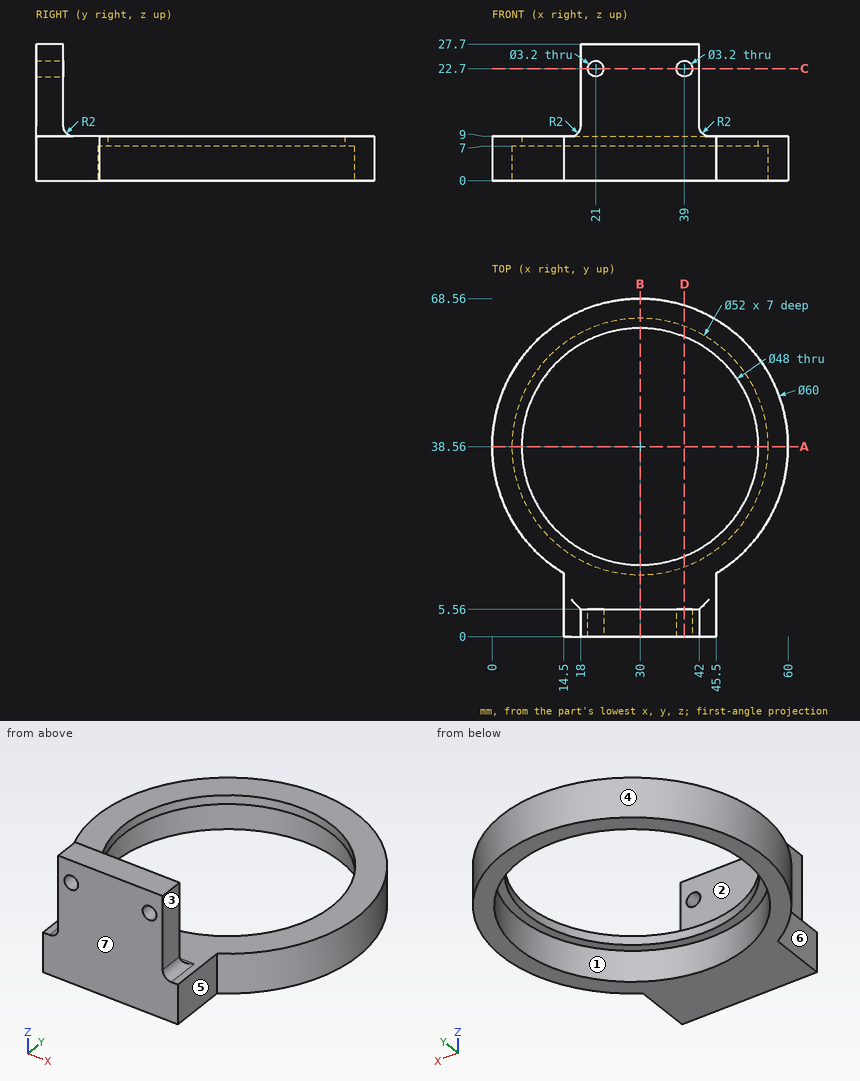
Study the drawing (mm; zero at the part's minimum x, y, z) and answer. A direction names the side the tool comes from. Give positions to 0.01 mm unless a question says otherwise; leave off trailing zeros. Write each loop counter-clockwise with the first axis right and the second up, starting at its lowest first coordinate (ties: lowest second). Pieces come first, ordered by that corner, then holes. Notation, with made-up numbers: (59, 78) -> (67, 78) arc R15 cw to (67, 105) -> close; hole circle Ø9 at (66.5, 70). An arc over 180 degrees is marked (long way). Answer as a JSON object with one key per item and string values. Group by question number.
1) Each of these flat-tipped pins is pushed along its axis until it touches: P1, Ø4.5, axis at y = 1.5, z = 20, coming from the +X side; P2, Ø7, axis at y = 8.5, z = 6, coming from the -X side; P3, Ø3, axis at y = 2.5, z = 19.5, coming from the -X side. Where does it stop, or does it pass through?
2) Find section B-B (x = 30). Write down the section's boundary in (y, z).
3) The mould has two halves that part along Y. Classify the marked faces 1, 2, 3 and 4: +Y half, -Y half, draft (parallel to the pull), parting line (faces both ways), or undercut.
4) Find section D-D (x = 39). Write down the section's boundary in (y, z), and give its area (3 significant figures).
5) Find section A-A (y = 38.56). Write down the section's boundary in (x, z), and give its area (3 significant figures).
6) Consider L1, parallel to X at y = 2.65, z = 22.7; L2, parallel to Z at x = 39, y = 3; L3, parallel to Y at x = 30, z = 3.75. Determine where each line is inside the solid, lowest interval first. Write a range as from..to.
7) A tool of negligible diameter and unlimited length cuts with its end or side. For the marked faces 5, 6 and 7, from which of +Z, -Z, +X, -X, +Y, -Y can it reach the whole face along a straight path? Write none if from no direction.
8) Find section C-C (z = 22.7). Write down the section's boundary in (x, y), and give its area (3 significant figures).
Values follow:
{
 "1": {"P1": "stops at x = 42", "P2": "stops at x = 14.5", "P3": "stops at x = 18"},
 "2": {"outline": "(0, 0) -> (12.56, 0) -> (12.56, 7) -> (14.56, 7) -> (14.56, 9) -> (7.56, 9) arc R2 cw to (5.56, 11) -> (5.56, 27.7) -> (0, 27.7) -> close; (62.56, 7) -> (64.56, 7) -> (64.56, 0) -> (68.56, 0) -> (68.56, 9) -> (62.56, 9) -> close"},
 "3": {"face 1": "undercut", "face 2": "+Y half", "face 3": "draft", "face 4": "parting line"},
 "4": {"outline": "(0, 0) -> (14.17, 0) -> (14.17, 7) -> (16.31, 7) -> (16.31, 9) -> (7.56, 9) arc R2 cw to (5.56, 11) -> (5.56, 21.1) -> (0, 21.1) -> close; (0, 24.3) -> (5.56, 24.3) -> (5.56, 27.7) -> (0, 27.7) -> close; (60.81, 7) -> (62.95, 7) -> (62.95, 0) -> (67.18, 0) -> (67.18, 9) -> (60.81, 9) -> close", "area": "261 mm2"},
 "5": {"outline": "(0, 0) -> (4, 0) -> (4, 7) -> (6, 7) -> (6, 9) -> (0, 9) -> close; (54, 7) -> (56, 7) -> (56, 0) -> (60, 0) -> (60, 9) -> (54, 9) -> close", "area": "80.0 mm2"},
 "6": {"L1": "x = 18..19.4, 22.6..37.4, 40.6..42", "L2": "z = 0..21.1, 24.3..27.7", "L3": "y = 0..12.56, 64.56..68.56"},
 "7": {"face 5": "+Z, -Z, +X, -Y", "face 6": "+Z, -Z, -X, -Y", "face 7": "+Z, -Z, +X, -X, -Y"},
 "8": {"outline": "(18, 0) -> (19.4, 0) -> (19.4, 5.56) -> (18, 5.56) -> close; (22.6, 0) -> (37.4, 0) -> (37.4, 5.56) -> (22.6, 5.56) -> close; (40.6, 0) -> (42, 0) -> (42, 5.56) -> (40.6, 5.56) -> close", "area": "97.9 mm2"}
}
